Build history of the part. All positions in model axes, mm. Give positions to 0.01 mm unless a question says otherwise; leave off trailing zeros. Order: outer loops, then holes, each group sorted by start corner. A loop starts at its lowest first (then second) coordinate and runs counter-clockwise, first axis right, second up. Notation, with made-up numbers: (9, -40) - (23, -40) arc R12 ccw to (23, -24) - close; hole circle Ø1 at (-0.75, 8). An arc over 180 degrees is marked (long way). Answer in a Markdown table with one row per item.
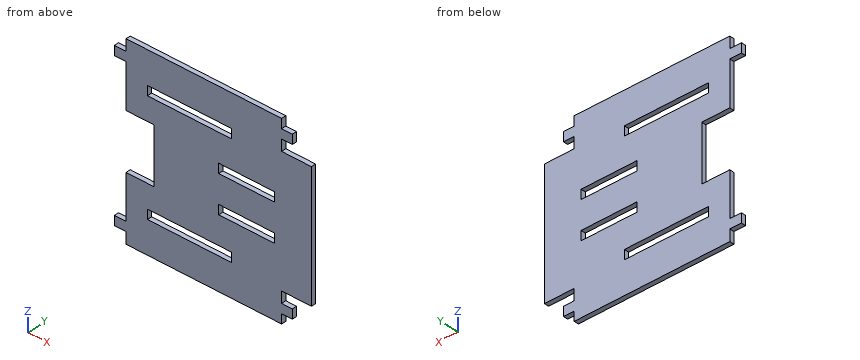
```python
from build123d import *

# Parameters (mm, degrees)
CROQUIS2_W              = 60
CROQUIS2_H              = 10
CROQUIS2_W_2            = 90
SALIENTE_EXTRUIR1_DEPTH = 5


with BuildPart() as part:
    # Croquis2 → Saliente-Extruir1 (new body)
    with BuildSketch(Plane(origin=(0, 0, 0), x_dir=(1, 0, 0), z_dir=(0, 1, 0))):
        Polygon((119.248757736, -67.751242264), (119.248757736, 67.751242264), (87.248757736, 67.751242264), (87.248757736, 79.751242264), (98.748757736, 79.751242264), (98.748757736, 89.751242264), (87.248757736, 89.751242264), (87.248757736, 99.751242264), (-79.502303886, 99.751242264), (-79.502303886, 87.5), (-92.002303886, 87.5), (-92.002303886, 77.5), (-79.502303886, 77.5), (-79.502303886, 30), (-49.502303886, 30), (-49.502303886, -30), (-79.502303886, -30), (-79.502303886, -77.5), (-92.002303886, -77.5), (-92.002303886, -87.5), (-79.502303886, -87.5), (-79.502303886, -99.751242264), (87.248757736, -99.751242264), (87.248757736, -89.751242264), (98.748757736, -89.751242264), (98.748757736, -79.751242264), (87.248757736, -79.751242264), (87.248757736, -67.751242264), align=None)
        with Locations((49.851646293, 20)):
            Rectangle(CROQUIS2_W, CROQUIS2_H, mode=Mode.SUBTRACT)
        with Locations((49.851646293, -20)):
            Rectangle(CROQUIS2_W, CROQUIS2_H, mode=Mode.SUBTRACT)
        with Locations((-11.573483533, -60)):
            Rectangle(CROQUIS2_W_2, CROQUIS2_H, mode=Mode.SUBTRACT)
        with Locations((-11.573483533, 60)):
            Rectangle(CROQUIS2_W_2, CROQUIS2_H, mode=Mode.SUBTRACT)
    extrude(amount=SALIENTE_EXTRUIR1_DEPTH)


solid = part.part
```
1. Cut at A-A on x = -77. Write the cut outline in (y, z), and give its area (3 significant figures).
Check result:
| item | result |
|---|---|
| outline | (0, -99.75) - (5, -99.75) - (5, -30) - (0, -30) - close; (0, 30) - (5, 30) - (5, 99.75) - (0, 99.75) - close |
| area | 698 mm² |
2. Cut at C-C on x = -34.5. Write the cut outline in (y, z).
Check result:
| item | result |
|---|---|
| outline | (0, -99.75) - (5, -99.75) - (5, -65) - (0, -65) - close; (0, -55) - (5, -55) - (5, 55) - (0, 55) - close; (0, 65) - (5, 65) - (5, 99.75) - (0, 99.75) - close |
3. Cut at B-B on z = 60.5. Write the cut outline in (x, y), and give its area (3 significant figures).
Check result:
| item | result |
|---|---|
| outline | (-79.5, 0) - (-56.57, 0) - (-56.57, 5) - (-79.5, 5) - close; (33.43, 0) - (119.25, 0) - (119.25, 5) - (33.43, 5) - close |
| area | 544 mm² |
4. Probe line 1 (Z direction, x = 3.5, y = 1.05); line 2 (Z direction, x = 20.5, y = 4.85); line 3 (Z direction, x = 57.5, y = 0.55). List the from-to ranges inside material, lowest first.
Check result:
| item | result |
|---|---|
| line 1 | z = -99.75 to -65, -55 to 55, 65 to 99.75 |
| line 2 | z = -99.75 to -65, -55 to -25, -15 to 15, 25 to 55, 65 to 99.75 |
| line 3 | z = -99.75 to -25, -15 to 15, 25 to 99.75 |
5. Drop flat-ended pins along their axis: P1, Ø2.5, axis at y = 3.5, z = -92.5, coming from the +X side; P2, Ø1.5, axis at y = 3.5, z = 60, coming from the -X side; P3, Ø1.5, axis at x = -87.5, y = 3, coming from the +Z side. Give the stop position or say it passes through.
Check result:
| item | result |
|---|---|
| P1 | stops at x = 87.25 |
| P2 | stops at x = -79.5 |
| P3 | stops at z = 87.5 |
6. Cut at D-D on y = 1.35. Count the separate pieces of the cut face and the enclosed holes in it, and give its area (3 significant figures).
Check result:
| item | result |
|---|---|
| separate pieces | 1 |
| enclosed holes | 4 |
| area | 33,300 mm² |
